Work out the finished part from the listing and answer in its coordinate system (mm). Face numbers are marked on the shaded views. A direction names the side the tool comes from. Round coordinates to 2 decimals unless told otherwise and drop trailing zeros. Loops run counter-clockwise (first coordinate to the right, second up) from the corner with the lowest first, then second, coordinate; pieces in that order, holes last.
```python
from build123d import *

# Parameters (mm, degrees)
F1_DEPTH = 18
F2_R     = 3


with BuildPart() as f1:
    # F0 (on Front) → F1 (new body)
    with BuildSketch(Plane.XZ):
        with BuildLine():
            ThreePointArc((-120, 5), (-118.535534, 1.464466), (-115, 0))
            Line((-115, 0), (-34.513279, 0))
            ThreePointArc((-34.513279, 0), (-8.382441, 9.715032), (5.055301, 34.141037))
            Line((5.055301, 34.141037), (16.844519, 113.759668))
            ThreePointArc((16.844519, 113.759668), (15.913712, 117.471576), (12.630817, 119.438111))
            Line((12.630817, 119.438111), (-3.196615, 121.781697))
            ThreePointArc((-3.196615, 121.781697), (-6.908523, 120.85089), (-8.875058, 117.567995))
            Line((-8.875058, 117.567995), (-20.664276, 37.949363))
            ThreePointArc((-20.664276, 37.949363), (-25.367486, 29.400261), (-34.513279, 26))
            Line((-34.513279, 26), (-115, 26))
            ThreePointArc((-115, 26), (-118.535534, 24.535534), (-120, 21))
            Line((-120, 21), (-120, 5))
        make_face()
    extrude(amount=F1_DEPTH)

    # F2
    f2_edges = [f1.edges().sort_by_distance(p)[0] for p in [
        (-14.769667, -18, 77.758679),
        (-25.367486, -18, 29.400261),
        (-74.75664, -18, 26),
        (-118.535534, -18, 24.535534),
        (-120, -18, 13),
        (-118.535534, -18, 1.464466),
        (-74.75664, -18, 0),
        (-8.382441, -18, 9.715032),
        (10.94991, -18, 73.950353),
        (15.913712, -18, 117.471576),
        (4.717101, -18, 120.609904),
        (-6.908523, -18, 120.85089),
        (-14.769667, 0, 77.758679),
        (-25.367486, 0, 29.400261),
        (-74.75664, 0, 26),
        (-118.535534, 0, 24.535534),
        (-120, 0, 13),
        (-118.535534, 0, 1.464466),
        (-74.75664, 0, 0),
        (-8.382441, 0, 9.715032),
        (10.94991, 0, 73.950353),
        (15.913712, 0, 117.471576),
        (4.717101, 0, 120.609904),
        (-6.908523, 0, 120.85089),
    ]]
    fillet(f2_edges, radius=F2_R)


solid = f1.part
```
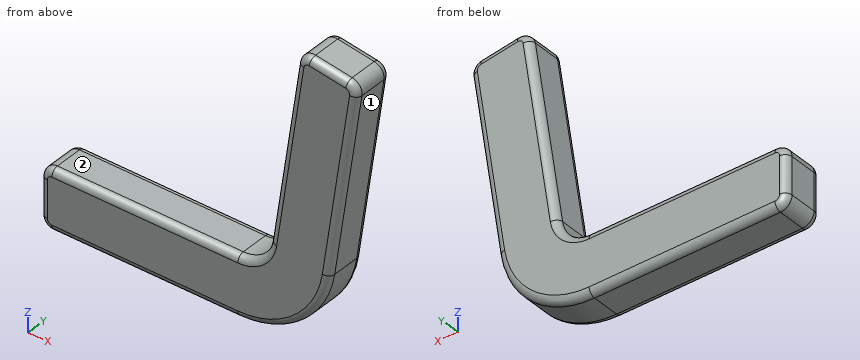
1. Find section A-A (y = -12.75). Write down the section's boundary in (x, z).
Answer key:
outline: (-120, 5) arc R5 ccw to (-115, 0) - (-34.51, 0) arc R40 ccw to (5.06, 34.14) - (16.84, 113.76) arc R5 ccw to (12.63, 119.44) - (-3.2, 121.78) arc R5 ccw to (-8.88, 117.57) - (-20.66, 37.95) arc R14 cw to (-34.51, 26) - (-115, 26) arc R5 ccw to (-120, 21) - close
2. Which of the six approach directions +Z, -Z, +X, -X, +Y, -Y give full straight-line access (tool end or side, diameter ignored) to the marked faces 1 and 2?
Answer key:
face 1: -Z, +X, +Y, -Y
face 2: +Z, -X, +Y, -Y
3. Consider probe 1 along Z at (x, y) = (-90, -9.75); probe 2 along X at (y, z) = (-10.5, 28); probe 3 along Z at (x, y) = (2, -6). Determine where each line is inside the solid, lowest interval first.
Answer key:
probe 1: z = 0 to 26
probe 2: x = -27.3 to 3.64
probe 3: z = 23.67 to 121.01
4. Find section B-B (x = -90.5). Write down the section's boundary in (y, z).
Answer key:
outline: (-18, 3) arc R3 ccw to (-15, 0) - (-3, 0) arc R3 ccw to (0, 3) - (0, 23) arc R3 ccw to (-3, 26) - (-15, 26) arc R3 ccw to (-18, 23) - close
5. Given pin 1 (5 mm diameter, centred on x = -75.5, y = -11.5, fed in from +Z); pin 2 (3 mm diameter, centred on y = -14.5, z = 37, fed in from -X); pin 3 (1 mm diameter, centred on y = -12.5, z = 34.5, fed in from +X); pin 4 (6 mm diameter, centred on x = -7, y = -5.5, fed in from +Z), each flat-ended and moving along its own axis, determine where each tip first touches the part or whether it passes through.
Answer key:
pin 1: stops at z = 26
pin 2: stops at x = -21.26
pin 3: stops at x = 5.18
pin 4: stops at z = 121.84
